Autodesk Inventor part; units mm, degrees
ref_plane "YZ Plane" through (0, 0, 0) normal (1, 0, 0) x (0, 1, 0)
ref_plane "XZ Plane" through (0, 0, 0) normal (0, 1, 0) x (-1, 0, 0)
ref_plane "XY Plane" through (0, 0, 0) normal (0, 0, 1) x (1, 0, 0)
sketch "Sketch1" plane through (0, 0, 0) normal (0, 0, 1) x (1, 0, 0)
  line L0 (12.7, 127) -> (12.7, -101.6)
  line L1 (12.7, -101.6) -> (-12.7, -101.6)
  line L2 (-12.7, -101.6) -> (-12.7, 127)
  arc A0 (88.9, 127) -> (12.7, 127) centre (50.8, 127) ccw
  arc A1 (114.3, 127) -> (-12.7, 127) centre (50.8, 127) ccw
  line L3 (88.9, 127) -> (114.3, 127)
  point P0 (0, 588.8574)
  point P1 (0, -101.6)
  dimension "d6" = 25.4
  dimension "d7" = 38.1
extrude "Extrusion1" add sketch "Sketch1" along normal blind 9.525
sketch "Sketch3" plane through (0, 0, 9.525) normal (0, 0, 1) x (1, 0, 0)
  line L0 (-12.7, 127) -> (-12.7, -101.6)
  line L1 (-12.7, -101.6) -> (12.7, -101.6)
  line L2 (12.7, -101.6) -> (12.7, 127)
  arc A0 (88.9, 127) -> (12.7, 127) centre (50.8, 127) ccw
  line L3 (88.9, 127) -> (114.3, 127)
  arc A1 (114.3, 127) -> (-12.7, 127) centre (50.8, 127) ccw
  point P0 (0, 0)
  point P1 (0, -76.2)
  dimension "d20" = 12.7
  dimension "d21" = 12.7
  dimension "d22" = 25.4
hole "Hole1" at (0, -76.2, 9.525) direction (0, 0, -1) diameter 6.7564 end through all
sketch "Sketch4" plane through (0, 0, 9.525) normal (0, 0, 1) x (1, 0, 0)
  circle A0 centre (0, -76.2) radius 3.3782
  line L0 (-12.7, 127) -> (-12.7, -101.6)
  line L1 (-12.7, -101.6) -> (12.7, -101.6)
  line L2 (12.7, -101.6) -> (12.7, 127)
  arc A1 (88.9, 127) -> (12.7, 127) centre (50.8, 127) ccw
  line L3 (88.9, 127) -> (114.3, 127)
  arc A2 (114.3, 127) -> (-12.7, 127) centre (50.8, 127) ccw
  line L4 (-3.3782, -25.4) -> (-3.3782, 25.4)
  line L5 (3.3782, 25.4) -> (3.3782, -25.4)
  circle A3 centre (0, -76.2) radius 3.3782
  arc A4 (3.3782, 25.4) -> (-3.3782, 25.4) centre (0, 25.4) ccw
  arc A5 (-3.3782, -25.4) -> (3.3782, -25.4) centre (0, -25.4) ccw
  point P0 (0, 0)
  dimension "d23" = 50.8
  dimension "d24" = 50.8
extrude "Extrusion2" cut sketch "Sketch4" against normal through all contours L4 A4 L5 A5
properties part number "ScissorHookTry"
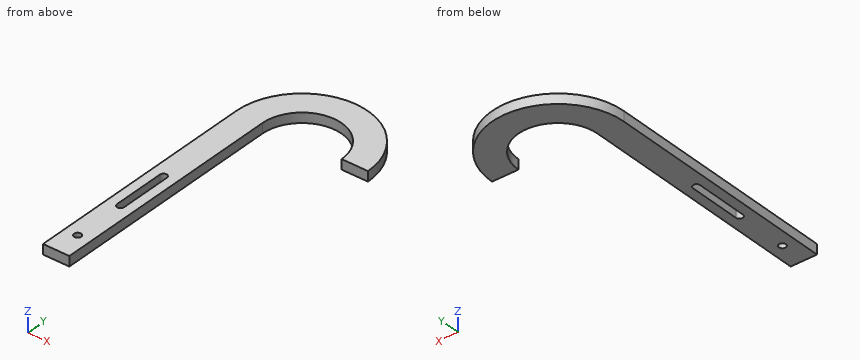
Geometry check sheet. Reference: the model listing, model coordinates, mm. Give positions to 0.01 mm unless a question says otherwise; leave off trailing zeros. Write each loop counter-clockwise with the first axis right and the second up, starting at its lowest first coordinate (ties: lowest second). Pieces come first, ordered by that corner, then holes.
1) Section check B-B, the plane z = 6. Record the boundary of the cut face in (x, y).
2) Section check A-A, the plane y = -76.2. Record the boundary of the cut face in (x, z) (3 decimals).
3) Section check D-D, the plane x = 50.8. Record the boundary of the cut face in (y, z) (3 decimals), and give its area (3 significant figures).
4) Material ranges on L1, parallel to Y at x = 0, z = 5; L2, parallel to X at y = -76.2, z = 2; L3, parallel to X at y = 98, z = 3.25, recorded low to high.
5) Section check C-C, the plane y = 115. Record the boundary of the cut face in (x, z) (3 decimals), and give its area (3 significant figures).
6) Gauge pin test, flat ends, axial feed: pin 1 (3 mm diameter, centred on y = 47, z = 3, fed in from +X); pin 2 (3 mm diameter, centred on x = 37.5, z = 5.5, fed in from +Y); pin 3 (4 mm diameter, centred on x = 70.5, z = 3, fed in from -Y). Record the tip position at first contact, or that the pin passes through.
Computed:
1. outline: (-12.7, -101.6) - (12.7, -101.6) - (12.7, 127) arc R38.1 cw to (88.9, 127) - (114.3, 127) arc R63.5 ccw to (-12.7, 127) - close; hole circle Ø6.76 at (0, -76.2); hole (-3.38, -25.4) arc R3.38 ccw to (3.38, -25.4) - (3.38, 25.4) arc R3.38 ccw to (-3.38, 25.4) - close
2. outline: (-12.7, 0) - (-3.378, 0) - (-3.378, 9.525) - (-12.7, 9.525) - close; (3.378, 0) - (12.7, 0) - (12.7, 9.525) - (3.378, 9.525) - close
3. outline: (165.1, 0) - (190.5, 0) - (190.5, 9.525) - (165.1, 9.525) - close
3. area: 242 mm2
4. L1: y = -101.6 to -79.58, -72.82 to -28.78, 28.78 to 165.1
4. L2: x = -12.7 to -3.38, 3.38 to 12.7
4. L3: x = -12.7 to 12.7
5. outline: (-12.7, 0) - (12.7, 0) - (12.7, 9.525) - (-12.7, 9.525) - close
5. area: 242 mm2
6. pin 1: stops at x = 12.7
6. pin 2: stops at y = 189.39
6. pin 3: stops at y = 158.32
